from build123d import *

# Parameters (mm, degrees)
SKETCH1_W           = 1057.275
SKETCH1_H           = 107.95
BOSS_EXTRUDE1_DEPTH = 76.2
SKETCH2_W           = 44.45
SKETCH2_H           = 76.2
BOSS_EXTRUDE2_DEPTH = 19.05
SKETCH3_R           = 6.35
CUT_EXTRUDE1_DEPTH  = 85.725
SKETCH4_W           = 3.175
SKETCH4_H           = 9.525
CUT_EXTRUDE2_DEPTH  = 1062.3906756
SKETCH5_R           = 12.7
CUT_EXTRUDE3_DEPTH  = 38.1


with BuildPart() as part:
    # Sketch1 → Boss-Extrude1 (new body)
    with BuildSketch(Plane.XY):
        Rectangle(SKETCH1_W, SKETCH1_H)
    extrude(amount=BOSS_EXTRUDE1_DEPTH)

    # Sketch2 → Boss-Extrude2 (add)
    with BuildSketch(Plane(origin=(528.6375, 0, 0), x_dir=(0, 0, -1), z_dir=(1, 0, 0))):
        with Locations((-38.1, 0)):
            Rectangle(SKETCH2_W, SKETCH2_H)
    boss_extrude2 = extrude(amount=BOSS_EXTRUDE2_DEPTH)

    # Sketch3 → Cut-Extrude1 (cut)
    with BuildSketch(Plane(origin=(547.6875, 0, 0), x_dir=(0, 0, -1), z_dir=(1, 0, 0))):
        with Locations((-25.4, 0)):
            Circle(SKETCH3_R)
    cut_extrude1 = extrude(amount=-CUT_EXTRUDE1_DEPTH, mode=Mode.SUBTRACT)

    # Sketch4 → Cut-Extrude2 (cut, through all)
    with BuildSketch(Plane(origin=(528.6375, 0, 0), x_dir=(0, 0, -1), z_dir=(1, 0, 0))):
        with Locations((-1.5875, 23.8125)):
            Rectangle(SKETCH4_W, SKETCH4_H)
    extrude(amount=-CUT_EXTRUDE2_DEPTH, mode=Mode.SUBTRACT)

    # Mirror1: Boss-Extrude2, Cut-Extrude1 across plane
    add(boss_extrude2.mirror(Plane(origin=(0, 0, 0), x_dir=(0, 0, 1), z_dir=(1, 0, 0))))
    add(cut_extrude1.mirror(Plane(origin=(0, 0, 0), x_dir=(0, 0, 1), z_dir=(1, 0, 0))), mode=Mode.SUBTRACT)

    # Sketch5 → Cut-Extrude3 (cut)
    with BuildSketch(Plane(origin=(0, 0, 0), x_dir=(-1, 0, 0), z_dir=(0, 0, -1))):
        with Locations((-461.9625, 0)):
            Circle(SKETCH5_R)
        with Locations((461.9625, 0)):
            Circle(SKETCH5_R)
    extrude(amount=-CUT_EXTRUDE3_DEPTH, mode=Mode.SUBTRACT)


solid = part.part
Geometry check sheet. Reference: the model listing, model coordinates, mm. A direction names the side the tool comes from. Coordinates: 2 decimals unless noted, no trailing zeros. Answer in a Markdown table with one row per item. Add a question column.
1) Gauge pin test, flat ends, axial feed: P1, Ø21, axis at x = -535, z = 32, coming from the +Y side (3 decimals); P2, Ø12.5, axis at x = -457.5, y = 1.5, coming from the -Z side; P3, Ø11.5, axis at y = 0, z = 25.4, coming from the +X side; P4, Ø10, axis at y = 0, z = 25.4, coming from the +X side. Record the tip position at first contact, or that the pin passes through.
2) Material ranges on line 1 along X through (y, z) = (-1, 6); line 2 along Y through (x, z) = (-497, 25.4) (3 decimals); line 3 along X through (y, z) = (-5.5, 34.5), recorded low to high. Write a range as [from, to].
3) Set-up check for faces 4 (the flat face through (-538, -1, 15.875)), 5 (the flat face through (538, -1, 15.875)), 6 (the flat face through (462, 0, 38.1)), 7 (the flat face through (-538, -1, 60.325)): record each of +Z, -Z, +X, -X, +Y, -Y from which the full face is reachable in a straight line by a thin tool's end or side.
4) Release check for a two-part mould opening along Y. For faces 1 (the flat face through (538, 38.1, 38)), 2 (the cylindrical face through (449.849, 3.815, 18.783)), 3 (the flat face through (-7, 41, 0)) record: +Y half, -Y half, draft (parallel to the pull), parting line (faces both ways), or undercut.
Check result:
| question | item | result |
|---|---|---|
| 1 | P1 | stops at y = 53.975 |
| 1 | P2 | stops at z = 38.1 |
| 1 | P3 | stops at x = 450.64 |
| 1 | P4 | stops at x = 450.29 |
| 2 | line 1 | x = [-528.64, -474.62], [-449.3, 449.3], [474.62, 528.64] |
| 2 | line 2 | y = [-53.975, -6.35], [6.35, 53.975] |
| 2 | line 3 | x = [-547.69, -473.41], [-450.52, 450.52], [473.41, 547.69] |
| 3 | face 4 | -Z, -X, +Y, -Y |
| 3 | face 5 | -Z, +X, +Y, -Y |
| 3 | face 6 | -Z |
| 3 | face 7 | +Z, -X, +Y, -Y |
| 4 | face 1 | +Y half |
| 4 | face 2 | undercut |
| 4 | face 3 | draft |
